For this review, take the finished solid that the model builds, in its own axes (mm). Coordinates: 2 decimals unless noted, no trailing zeros. Order: outer loops, then holes, each group sorted by start corner. A loop starts at its lowest first (then second) coordinate and runs counter-clockwise, first axis right, second up. Notation, with made-up numbers: (-40, 7) - (-29, 7) arc R28 cw to (-29, 28) - close; hole circle Ø8 at (84.5, -20). An arc over 180 degrees is marked (long way). One line per item, written item: value. Start each with the question number.
(1) Clearance check with flat-ended pins moving along their axes: pin 1 (4.5 mm diameter, centred on x = 5, y = 5, fed in from -Z); pin 2 (1.5 mm diameter, centred on y = 1.5, z = -1, fed in from +X). State where each tip first meets the part, or that it passes through.
(2) Consider section B-B on y = 5. Write out the cut boundary in (x, z) (3 decimals).
(3) Mouldability with a two-part tool opening along Y and no side actions: class faces 1 (the cylindrical face through (50.63, 4.22, -2.54)), 2 (the flat face through (28, 0, -3)), 3 (the cylindrical face through (6.61, 3.77, -2.54)), 4 (the flat face through (28, 10, -3)) as released by +Y, released by -Y, zero draft, split by the parting line, or undercut.
(4) Consider section A-A on x = 5. Write out the cut boundary in (y, z) (3 decimals).
(5) Consider section D-D on y = 8.75. Write out the cut boundary in (x, z).
(6) To check wall thickness, follow line 1 along Y through (x, z) = (5, -1.3) (3 decimals); line 2 along X through (y, z) = (5.25, -1.6); line 3 along X through (y, z) = (2.75, -4.6). State the ranges of each line that lie inside material, in increasing order.
(7) Consider section C-C on z = -3.45. Write out the cut boundary in (x, y) (3 decimals), then the cut area to 3 significant figures.
```python
from build123d import *

# Parameters (mm, degrees)
SKETCH_5_W          = 57.5
SKETCH_5_H          = 5
EXTRUDE_3_DEPTH     = 10
SKETCH_6_R          = 2.025
CUT_EXTRUDE_4_DEPTH = 59.576872569
FILLET_4_R          = 3


with BuildPart() as part:
    # 草图5 → 凸台-拉伸3 (new body)
    with BuildSketch(Plane(origin=(0, 0, 0), x_dir=(1, 0, 0), z_dir=(0, 1, 0))):
        with Locations((28.75, 2.5)):
            Rectangle(SKETCH_5_W, SKETCH_5_H)
    extrude(amount=EXTRUDE_3_DEPTH)

    # 草图6 → 切除-拉伸4 (cut, through all)
    with BuildSketch(Plane(origin=(0, 0, -5), x_dir=(-1, 0, 0), z_dir=(0, 0, -1))):
        with Locations((-52.5, 5)):
            Circle(SKETCH_6_R)
        with Locations((-5, 5)):
            Circle(SKETCH_6_R)
    extrude(amount=-CUT_EXTRUDE_4_DEPTH, mode=Mode.SUBTRACT)

    # 圆角4
    fillet_4_edges = [part.edges().sort_by_distance(p)[0] for p in [
        (57.5, 10, -2.5),
        (0, 10, -2.5),
        (57.5, 0, -2.5),
        (0, 0, -2.5),
    ]]
    fillet(fillet_4_edges, radius=FILLET_4_R)


solid = part.part
```
Geometry check:
1. pin 1: stops at z = -5
1. pin 2: stops at x = 57.4
2. outline: (0, -5) - (2.975, -5) - (2.975, 0) - (0, 0) - close; (7.025, -5) - (50.475, -5) - (50.475, 0) - (7.025, 0) - close; (54.525, -5) - (57.5, -5) - (57.5, 0) - (54.525, 0) - close
3. face 1: undercut
3. face 2: released by -Y
3. face 3: undercut
3. face 4: released by +Y
4. outline: (0, -5) - (2.975, -5) - (2.975, 0) - (0, 0) - close; (7.025, -5) - (10, -5) - (10, 0) - (7.025, 0) - close
5. outline: (0.56, -5) - (56.94, -5) - (56.94, 0) - (0.56, 0) - close
6. line 1: y = 0 to 2.975, 7.025 to 10
6. line 2: x = 0 to 2.99, 7.01 to 50.49, 54.51 to 57.5
6. line 3: x = 0.01 to 57.49
7. outline: (0, 3) arc R3 ccw to (3, 0) - (54.5, 0) arc R3 ccw to (57.5, 3) - (57.5, 7) arc R3 ccw to (54.5, 10) - (3, 10) arc R3 ccw to (0, 7) - close; hole circle Ø4.05 at (5, 5); hole circle Ø4.05 at (52.5, 5)
7. area: 542 mm^2
